Input: dimensioned drawing with shaded views. Units: mm. Origin: part minimum x, y, z. A direction names the side the tool comes from. Round coordinates to 2 decimals unless told otherwise and drop trailing zeros. Order: outer loops, then holes, each group sorted by start corner. A loop starts at its lowest first (then second) coordinate and runs counter-clockwise, first axis right, second up. Notation, with made-up numbers: (60.5, 49) - (102.5, 49) arc R30 cw to (102.5, 80) - close; hole circle Ø11 at (40, 7). An arc over 180 degrees is marked (long way). One line per item, written item: value. Start each with the question number.
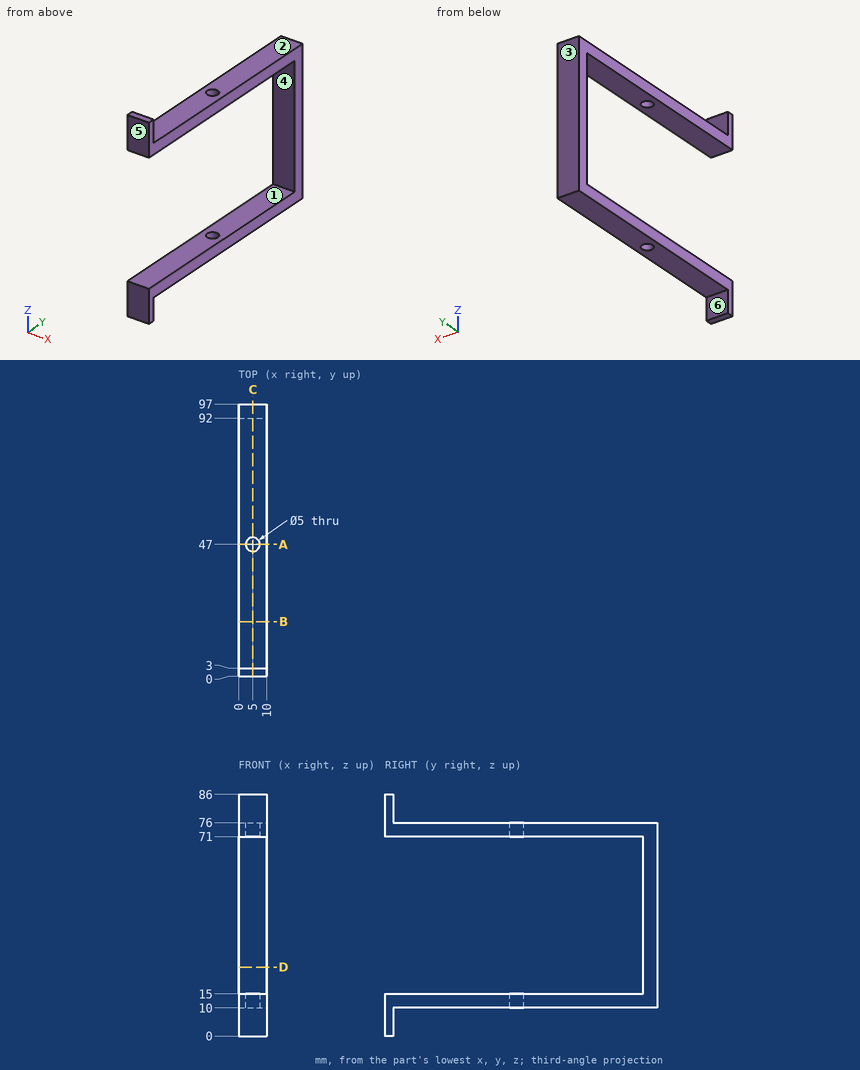
1. Section A-A (y = 47). Return the cut outline in (x, z).
2. Section B-B (y = 19.5). Return the cut outline in (x, z).
3. Line query: line 1 (Z direction, x = 9.25, y = 9.5); line 2 (Y direction, x = 5, z = 72.85); line 3 (Y direction, x = 4.75, z = 54). Output: solid intervals per line, ascending. Write a range as from..to.
4. Set-up query: the marked faces 4, 5 and 6. Return all of +Z, -Z, +X, -X, +Y, -Y with unobstructed straight access to the full face (end or side cutting, diameter ignored); none if empty.
5. Pin query (flat end, axial travel): pin 1 (5 mm diameter, centred on x = 5, z = 18, fed in from -Y); pin 2 (3 mm diameter, centred on x = 4.5, z = 4, fed in from +Y); pin 3 (3 mm diameter, centred on x = 7, y = 39.5, fed in from +Z); pin 4 (10 mm diameter, centred on y = 23.5, z = 9.5, fed in from -X). Return the tip coordinate at first contact, or that it passes through.
6. Pull-direction query (Z, two-part tool) for the marked faces 1, 2 and 3; classes: released by +Z, released by -Z, zero draft, split by the parting line, or undercut.
7. Section C-C (x = 5). Return the cut outline in (y, z), then the cut area to 3 significant figures.
8. Section D-D (z = 24.5). Return the cut outline in (x, y), then the cut area to 3 significant figures.
Solved:
1. outline: (0, 10) - (2.5, 10) - (2.5, 15) - (0, 15) - close; (0, 71) - (2.5, 71) - (2.5, 76) - (0, 76) - close; (7.5, 10) - (10, 10) - (10, 15) - (7.5, 15) - close; (7.5, 71) - (10, 71) - (10, 76) - (7.5, 76) - close
2. outline: (0, 10) - (10, 10) - (10, 15) - (0, 15) - close; (0, 71) - (10, 71) - (10, 76) - (0, 76) - close
3. line 1: z = 10..15, 71..76
3. line 2: y = 0..44.5, 49.5..97
3. line 3: y = 92..97
4. face 4: +X, -X, -Y
4. face 5: +Z, -Z, +X, -X, -Y
4. face 6: -Z, +X, -X, +Y
5. pin 1: stops at y = 92
5. pin 2: stops at y = 3
5. pin 3: stops at z = 76
5. pin 4: stops at x = 0
6. face 1: undercut
6. face 2: released by +Z
6. face 3: zero draft
7. outline: (0, 0) - (3, 0) - (3, 10) - (44.5, 10) - (44.5, 15) - (0, 15) - close; (0, 71) - (44.5, 71) - (44.5, 76) - (3, 76) - (3, 86) - (0, 86) - close; (49.5, 10) - (97, 10) - (97, 76) - (49.5, 76) - (49.5, 71) - (92, 71) - (92, 15) - (49.5, 15) - close
7. area: 1,260 mm²
8. outline: (0, 92) - (10, 92) - (10, 97) - (0, 97) - close
8. area: 50.0 mm²
